CAD build for the part. Positions are in the model's coordinates, mm. Face numbers are marked on the shaded views. A direction names the side the tool comes from. Give positions to 0.01 mm unless a question says otherwise; leave off trailing zeros. Write each loop counter-clockwise with the first axis right and the second up, starting at its lowest first coordinate (ties: lowest second). Pieces come first, ordered by that corner, then holes. Notation, with made-up numbers: (67, 70.5) - (86, 70.5) arc R11 ccw to (86, 78.5) - close; hole circle Ø7 at (57, -32). An arc over 180 degrees is marked (long way). Answer as a JSON object with one key per item and string values.
from build123d import *

# Parameters (mm, degrees)
SKETCH_W           = 6.3
SKETCH_H           = 1
PAD_DEPTH          = 4
POLARPATTERN_COUNT = 12
CYLINDER002_R      = 2.4
CYLINDER002_DEPTH  = 6


with BuildPart() as obj1:
    # Sketch → Pad (new body)
    with BuildSketch(Plane.XY):
        with Locations((-3.15, 0)):
            Rectangle(SKETCH_W, SKETCH_H)
    pad = extrude(amount=PAD_DEPTH)

    # PolarPattern: Pad ×12 about axis
    polarpattern_axis = Axis((0, 0, 0), (0, 0, 1))
    for i in range(1, POLARPATTERN_COUNT):
        add(pad.rotate(polarpattern_axis, i * 360 / POLARPATTERN_COUNT))


with BuildPart() as obj1_1:
    # Body placement: moved
    add(obj1.part.moved(Location((0, 0, 2))))


with BuildPart() as obj2:
    # Cylinder002 → Cylinder002 (new body)
    with BuildSketch(Plane.XY):
        Circle(CYLINDER002_R)
    extrude(amount=CYLINDER002_DEPTH)

    # Fusion: union obj1
    add(obj1_1.part)


solid = obj2.part
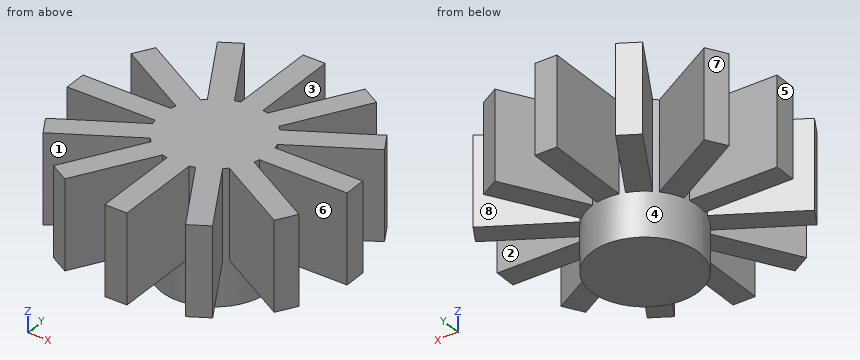
(1) 3-axis set-ups, long thin cutter, end or side, ignore diameter. For the marked faces 1, 2, 3 and 4: which of +Z, -Z, +X, -X, +Y, -Y reach the whole face in a straight line?
Answer key:
{"face 1": "+Z, -Z", "face 2": "+Z, -Z, +X", "face 3": "+Z, -Z, +Y", "face 4": "-Z"}
(2) Pull direction Y, two halves, no side cores. Call the marked faces 5, 6, 7 and 8: pulls with the +Y half, pulls with the -Y half, needs draft (parallel to the pull), parting line crosses it, or undercut.
Answer key:
{"face 5": "needs draft", "face 6": "undercut", "face 7": "pulls with the +Y half", "face 8": "undercut"}
(3) Saw through at A-A, the plane y = 0. Give the cut face in (x, z), and give its area (3 significant figures).
Answer key:
{"outline": "(-6.3, 2) - (-2.4, 2) - (-2.4, 0) - (2.4, 0) - (2.4, 2) - (6.3, 2) - (6.3, 6) - (-6.3, 6) - close", "area": "60.0 mm²"}
(4) Flat gauge pins, fed straight in: P1, Ø2, axis at x = -4.5, z = 5, coming from the -Y side; P2, Ø3, axis at y = 4.5, z = 5, coming from the -X side; P3, Ø2, axis at y = -5, z = 3.5, coming from the +X side; P4, Ø6, axis at x = -1.5, y = -4, coming from the -Z side. Where does each tip first touch, or does it go through?
Answer key:
{"P1": "stops at y = -5.25", "P2": "stops at x = -5.54", "P3": "stops at x = 3.58", "P4": "stops at z = 0"}
(5) Saw through at D-D, the plane x = 4.25. Give the cut face in (y, z), and give its area (3 significant figures).
Answer key:
{"outline": "(-3.03, 2) - (-1.88, 2) - (-1.88, 6) - (-3.03, 6) - close; (-0.5, 2) - (0.5, 2) - (0.5, 6) - (-0.5, 6) - close; (1.88, 2) - (3.03, 2) - (3.03, 6) - (1.88, 6) - close", "area": "13.2 mm²"}
(6) Saw through at C-C, the plane y = 2. Give the cut face in (x, z), and give its area (3 significant figures).
Answer key:
{"outline": "(-4.46, 2) - (-2.46, 2) - (-2.46, 6) - (-4.46, 6) - close; (-1.73, 2) - (-1.33, 2) - (-1.33, 0) - (1.33, 0) - (1.33, 2) - (1.73, 2) - (1.73, 6) - (-1.73, 6) - close; (2.46, 2) - (4.46, 2) - (4.46, 6) - (2.46, 6) - close", "area": "35.2 mm²"}
(7) Probe L1, parallel to Y at x = 4.75, z = 3.3; L2, parallel to X at y = 2.75, z = 4.85; L3, parallel to Y at x = -5, z = 2.45. List the from-to ranges inside material, lowest first. Write a range as [from, to].
Answer key:
{"L1": "y = [-3.32, -2.17], [-0.5, 0.5], [2.17, 3.32]", "L2": "x = [-5.69, -3.76], [-2.17, -1.01], [-0.5, 0.5], [1.01, 2.17], [3.76, 5.69]", "L3": "y = [-3.46, -2.31], [-0.5, 0.5], [2.31, 3.46]"}
